Model file for the job. Use its own axes, mm. Face numbers are marked on the shaded views. A direction names the side the tool comes from. Round coordinates to 2 decimals unless told otherwise and drop trailing zeros. Loops run counter-clockwise (first coordinate to the right, second up) from the corner with the lowest first, then second, coordinate; pieces in that order, holes last. Notation, with made-up numbers: (-28, 22) -> (10, 22) arc R30 cw to (10, 53) -> close; hole circle Ø2 at (-26.75, 58). An arc over 180 degrees is marked (long way). Use a Markdown table: item, result.
from build123d import *

# Parameters (mm, degrees)
CROQUIS1_R              = 19.3
CROQUIS1_R_2            = 1.6
SALIENTE_EXTRUIR1_DEPTH = 1.5
CROQUIS2_R              = 12
CROQUIS2_R_2            = 1.6
CORTAR_EXTRUIR1_DEPTH   = 2


with BuildPart() as part:
    # Croquis1 → Saliente-Extruir1 (new, symmetric)
    with BuildSketch(Plane.XY):
        Circle(CROQUIS1_R)
        with Locations((0, 16)):
            Circle(CROQUIS1_R_2, mode=Mode.SUBTRACT)
        Circle(CROQUIS1_R_2, mode=Mode.SUBTRACT)
        with Locations((13.856406461, 8)):
            Circle(CROQUIS1_R_2, mode=Mode.SUBTRACT)
        with Locations((13.856406461, -8)):
            Circle(CROQUIS1_R_2, mode=Mode.SUBTRACT)
        with Locations((0, -16)):
            Circle(CROQUIS1_R_2, mode=Mode.SUBTRACT)
        with Locations((-13.856406461, -8)):
            Circle(CROQUIS1_R_2, mode=Mode.SUBTRACT)
        with Locations((-13.856406461, 8)):
            Circle(CROQUIS1_R_2, mode=Mode.SUBTRACT)
    extrude(amount=SALIENTE_EXTRUIR1_DEPTH, both=True)

    # Croquis2 → Cortar-Extruir1 (cut)
    with BuildSketch(Plane(origin=(0, 0, -1.5), x_dir=(-1, 0, 0), z_dir=(0, 0, -1))):
        Circle(CROQUIS2_R)
        Circle(CROQUIS2_R_2, mode=Mode.SUBTRACT)
    extrude(amount=-CORTAR_EXTRUIR1_DEPTH, mode=Mode.SUBTRACT)


solid = part.part
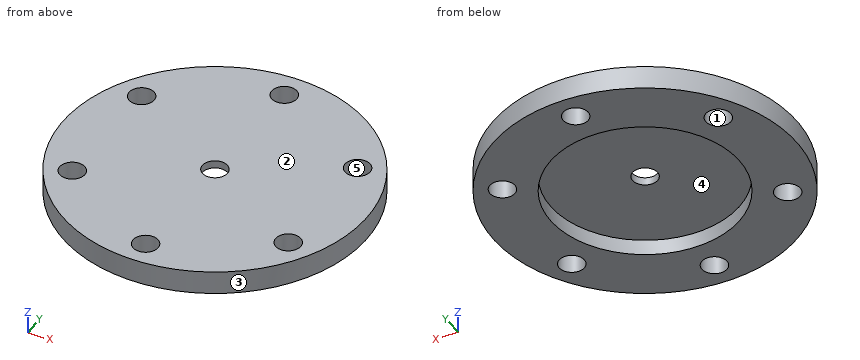
Q1. Flat gauge pins, fed straight in: pin 1 (3 mm diameter, centred on x = 0, y = 0, fed in from -Z); pin 2 (1 mm diameter, centred on x = 8.5, y = 3, fed in from -Z). Where does each tip first touch, or does it go through?
Results list:
| item | result |
|---|---|
| pin 1 | passes through |
| pin 2 | stops at z = 0.5 |
Q2. Band-saw the part on C-C, the plane y = -16. Give the cut face in (x, z).
Results list:
| item | result |
|---|---|
| outline | (-10.79, -1.5) -> (-1.6, -1.5) -> (-1.6, 1.5) -> (-10.79, 1.5) -> close; (1.6, -1.5) -> (10.79, -1.5) -> (10.79, 1.5) -> (1.6, 1.5) -> close |
Q3. Band-saw the part on B-B, the plane z = -0.5. Give the cut face in (x, y).
Results list:
| item | result |
|---|---|
| outline | circle Ø38.6 at (0, 0); hole circle Ø3.2 at (-13.86, -8); hole circle Ø3.2 at (-13.86, 8); hole circle Ø24 at (0, 0); hole circle Ø3.2 at (0, -16); hole circle Ø3.2 at (0, 16); hole circle Ø3.2 at (13.86, -8); hole circle Ø3.2 at (13.86, 8) |
Q4. Drill centre lines: L1, parallel to Y at x = -13.5, z = 0.4; L2, parallel to Y at x = 0, z = -0.8; L3, parallel to Y at x = -12.5, z = -0.7. Where is each one in solid material? Low to high. Write a range as from..to.
Results list:
| item | result |
|---|---|
| L1 | y = -13.79..-9.56, -6.44..6.44, 9.56..13.79 |
| L2 | y = -19.3..-17.6, -14.4..-12, 12..14.4, 17.6..19.3 |
| L3 | y = -14.71..-8.85, -7.15..7.15, 8.85..14.71 |
Q5. Tool access for the marked faces 4 and 5: list every direction of +Z, -Z, +X, -X, +Y, -Y with a clear straight run to the whole face (end or side of a thin tool).
Results list:
| item | result |
|---|---|
| face 4 | -Z |
| face 5 | +Z, -Z |
Q6. Pull direction Y, two halves, no side cores. Call the marked faces 1, 2 and 3: released by +Y, released by -Y, zero draft, split by the parting line, or undercut.
Results list:
| item | result |
|---|---|
| face 1 | undercut |
| face 2 | zero draft |
| face 3 | split by the parting line |
Q7. Band-saw the part on D-D, the plane x = -14. Give the cut face in (y, z), plus the area to 3 significant figures.
Results list:
| item | result |
|---|---|
| outline | (-13.28, -1.5) -> (-9.59, -1.5) -> (-9.59, 1.5) -> (-13.28, 1.5) -> close; (-6.41, -1.5) -> (6.41, -1.5) -> (6.41, 1.5) -> (-6.41, 1.5) -> close; (9.59, -1.5) -> (13.28, -1.5) -> (13.28, 1.5) -> (9.59, 1.5) -> close |
| area | 60.6 mm² |
Q8. Band-saw the part on A-A, the plane x = 0. Give the cut face in (y, z).
Results list:
| item | result |
|---|---|
| outline | (-19.3, -1.5) -> (-17.6, -1.5) -> (-17.6, 1.5) -> (-19.3, 1.5) -> close; (-14.4, -1.5) -> (-12, -1.5) -> (-12, 0.5) -> (-1.6, 0.5) -> (-1.6, 1.5) -> (-14.4, 1.5) -> close; (1.6, 0.5) -> (12, 0.5) -> (12, -1.5) -> (14.4, -1.5) -> (14.4, 1.5) -> (1.6, 1.5) -> close; (17.6, -1.5) -> (19.3, -1.5) -> (19.3, 1.5) -> (17.6, 1.5) -> close |
